The listing builds one solid part. Answer for the finished solid, in the listing's coordinates (mm). A direction names the side the tool comes from. Give positions to 0.01 mm unless a question says otherwise; leave off trailing zeros. Order: outer loops, then holes, each group sorted by start corner. A loop starts at its lowest first (then second) coordinate and runs counter-clockwise, first axis right, second up. Notation, with made-up numbers: (41.25, 39) - (97.25, 39) arc R17 ccw to (97.25, 54) - close; hole circle Ø6 at (88, 53). An arc over 180 degrees is marked (long way). Use a Markdown table: item, result. Add a question column.
1) Flat-ended cylindrical pins translate along their axes: pin 1 (1.5 mm diameter, centred on y = 1, z = -10, fed in from -X); pin 2 (1.8 mm diameter, centred on y = -0.5, z = -13, fed in from +X). Find the tip coordinate at first contact, or state that the pin passes through.
2) Find section A-A, the plane z = -7. Determine the outline of the cut face in (x, y), plus the area to 3 significant figures.
3) Straight lines are drawn through the part: line 1 (Y direction, x = 2.55, z = -1.25); line 2 (X direction, y = -0.65, z = -1); line 3 (Y direction, x = 0.85, z = 2.5). For each, find the intervals that lie inside material, in ascending order.
4) For faces 1 (the face through (1.287, 0, -13)), 2 (the face through (1.847, -0.27, -9.573)), determine the directions among +Z, -Z, +X, -X, +Y, -Y from which every point of the face is accessible in a straight line to the end or side of a thin tool.
5) The mould has two halves that part along Z. Classify faces 3 (the face through (1.28, -0.09, 3.54)), 4 (the face through (0.664, 0, -13)), 5 (the face through (1, 0, -14.636)): released by +Z, released by -Z, zero draft, split by the parting line, or undercut.
from build123d import *

# Parameters (mm, degrees)
F2_W     = 0.6228546263
F2_H     = 2.4024397135
F3_DEPTH = 12.7
F4_R     = 5.08


with BuildPart() as f1:
    # F0 (on Front) → F1 (revolve)
    with BuildSketch(Plane.XZ):
        with BuildLine():
            Line((1.8883474847, 0), (0.9883474847, 5.3636118397))
            Line((0.9883474847, 5.3636118397), (0.9883474847, -14.6363881603))
            Line((0.9883474847, -14.6363881603), (1.8883474847, -14.6363881603))
            Line((1.8883474847, -14.6363881603), (1.8883474847, -2.6669100628))
            ThreePointArc((1.8883474847, -2.6669100628), (2.7959176273, -1.3334550314), (1.8883474847, 0))
        make_face()
    revolve(axis=Axis((0.9883474847, 0, -4.6363881603), (0, 0, -1)))

    # F2 (on Front) → F3 (cut, symmetric)
    with BuildSketch(Plane.XZ):
        with Locations((0.9755069332, -12.7969710156)):
            Rectangle(F2_W, F2_H)
    extrude(amount=F3_DEPTH, both=True, mode=Mode.SUBTRACT)

    # F4
    f4_edges = [f1.edges().sort_by_distance(p)[0] for p in [
        (0.088347, 0, -2.66691),
        (0.088347, 0, 0),
    ]]
    fillet(f4_edges, radius=F4_R)


solid = f1.part
The answers:
| question | item | result |
|---|---|---|
| 1 | pin 1 | x = 0.12 |
| 1 | pin 2 | x = 1.89 |
| 2 | outline | circle Ø1.8 at (0.99, 0) |
| 2 | area | 2.54 mm2 |
| 3 | line 1 | -0.91 to 0.91 |
| 3 | line 2 | -0.66 to 2.63 |
| 3 | line 3 | -0.46 to 0.46 |
| 4 | face 1 | +Y, -Y |
| 4 | face 2 | -Z |
| 5 | face 3 | released by +Z |
| 5 | face 4 | undercut |
| 5 | face 5 | released by -Z |
